Verification items for the finished model (mm, model axes). Give positions to 0.01 mm unless a question says otherwise; leave off trailing zeros. Loops run counter-clockwise (first coordinate to the right, second up) from the corner with the lowest first, then second, coordinate; pieces in that order, holes last. Notation, with made-up numbers: (51, -1) - (102, -1) arc R29 ccw to (102, 29) - close; hole circle Ø3 at (44.25, 49.25). An arc over 180 degrees is marked (long way). One line per question, with ' | ' between items. Start each with the question number.
1. Section check B-B, the plane y = 119.25. Enter the section's corners in (x, z) (3 decimals), then the cut area to 3 significant figures.
2. Thickness scan on line 1 along X through (y, z) = (122.25, 275) (3 decimals); line 2 along Z through (x, y) = (2300, 122) (3 decimals); line 3 along X through (y, z) = (123.5, 283). Record the ranges inside material, lowest first. Write a range as from..to.
3. Section check A-A, the plane z = 275. Enter the section's corners in (x, y) (3 decimals).
4. Section check C-C, the plane x = 2600. Enter the section's corners in (y, z) (3 decimals), then the cut area to 3 significant figures.
from build123d import *

# Parameters (mm, degrees)
BOSS_EXTRUDE1_DEPTH      = 50.8
BOSS_EXTRUDE1_DEPTH_BACK = 38.1
SKETCH2_W                = 381
SKETCH2_H                = 12.7
SKETCH3_W                = 12.7
SKETCH3_H                = 44.45
CUT_EXTRUDE1_DEPTH       = 2664.230012597
CAVITY1_START            = 115.8
CAVITY1_OUTLINE_R        = 12.7
CAVITY1_DEPTH            = 12.7
MOVE_FACE_HOLES_BY       = 0.635
MOVE_FACE_HOLES_2_BY     = 0.635
MOVE_FACE2_BY            = 0.762
MOVE_FACE2_2_BY          = 0.762
MOVE_FACE2_3_BY          = 0.762
SLOT_FILLET_R            = 3.175


# Read off the part's stored shape, not the designer's step: Cavity1
with BuildPart() as part:
    # Sketch2 → Boss-Extrude1 (new, two sides: drawn at the far end of the back side and taken through both)
    with BuildSketch(Plane.XY.offset(287.7).offset(-BOSS_EXTRUDE1_DEPTH_BACK)):
        with Locations((2451.1, 122.15)):
            Rectangle(SKETCH2_W, SKETCH2_H)
    extrude(amount=BOSS_EXTRUDE1_DEPTH + BOSS_EXTRUDE1_DEPTH_BACK)

    # Sketch3 → Cut-Extrude1 (cut, through all)
    with BuildSketch(Plane(origin=(0, 128.5, 0), x_dir=(1, 0, 0), z_dir=(0, 1, 0))):
        with Locations((2470.15, -271.825)):
            Rectangle(SKETCH3_W, SKETCH3_H)
    extrude(amount=-CUT_EXTRUDE1_DEPTH, mode=Mode.SUBTRACT)

    # Cavity1 outline → Cavity1 (cut)
    with BuildSketch(Plane(origin=(0, 0, 0), x_dir=(1, 0, 0), z_dir=(0, 1, 0)).offset(CAVITY1_START)):
        with Locations((2300, -275)):
            Circle(CAVITY1_OUTLINE_R)
        with Locations((2600, -275)):
            Circle(CAVITY1_OUTLINE_R)
    extrude(amount=CAVITY1_DEPTH, mode=Mode.SUBTRACT)

    # Move Face Holes: a curved face moved outward by 0.635
    add(Solid.thicken(part.faces().sort_by_distance((2587.3, 122.15, 275))[0], MOVE_FACE_HOLES_BY))

    # Move Face Holes 2: a curved face moved outward by 0.635
    add(Solid.thicken(part.faces().sort_by_distance((2287.3, 122.15, 275))[0], MOVE_FACE_HOLES_2_BY))

    # Move Face2: a face moved inward by 0.762
    extrude(part.faces().sort_by_distance((2470.15, 122.15, 294.05))[0], amount=MOVE_FACE2_BY, dir=(0, 0, 1), mode=Mode.SUBTRACT)

    # Move Face2 2: a face moved inward by 0.762
    extrude(part.faces().sort_by_distance((2476.5, 122.15, 271.825))[0], amount=MOVE_FACE2_2_BY, dir=(1, 0, 0), mode=Mode.SUBTRACT)

    # Move Face2 3: a face moved inward by 0.762
    extrude(part.faces().sort_by_distance((2463.8, 122.15, 271.825))[0], amount=MOVE_FACE2_3_BY, dir=(-1, 0, 0), mode=Mode.SUBTRACT)

    # Slot Fillet
    slot_fillet_edges = [part.edges().sort_by_distance(p)[0] for p in [
        (2477.262, 122.15, 294.812),
        (2463.038, 122.15, 294.812),
    ]]
    fillet(slot_fillet_edges, radius=SLOT_FILLET_R)


solid = part.part
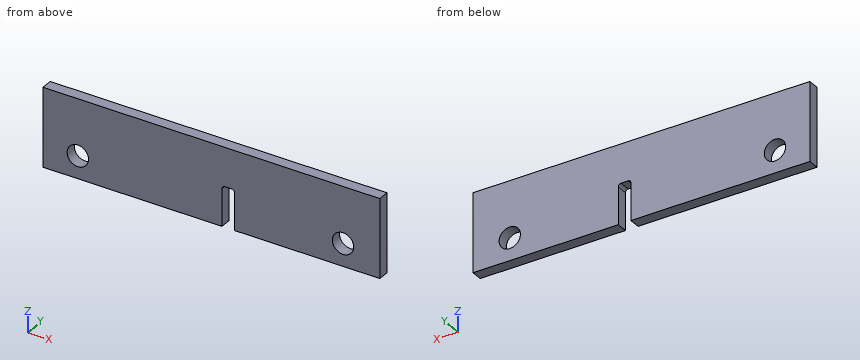
Results list:
1) outline: (2260.6, 249.6) - (2463.038, 249.6) - (2463.038, 291.637) arc R3.175 cw to (2466.213, 294.812) - (2474.087, 294.812) arc R3.175 cw to (2477.262, 291.637) - (2477.262, 249.6) - (2641.6, 249.6) - (2641.6, 338.5) - (2260.6, 338.5) - close; hole circle Ø24.13 at (2300, 275); hole circle Ø24.13 at (2600, 275) | area: 32,300 mm²
2) line 1: 2260.6..2287.935, 2312.065..2463.038, 2477.262..2587.935, 2612.065..2641.6 | line 2: 249.6..262.935, 287.065..338.5 | line 3: 2260.6..2290.97, 2309.03..2463.04, 2477.26..2590.97, 2609.03..2641.6
3) outline: (2260.6, 115.8) - (2287.935, 115.8) - (2287.935, 128.5) - (2260.6, 128.5) - close; (2312.065, 115.8) - (2463.038, 115.8) - (2463.038, 128.5) - (2312.065, 128.5) - close; (2477.262, 115.8) - (2587.935, 115.8) - (2587.935, 128.5) - (2477.262, 128.5) - close; (2612.065, 115.8) - (2641.6, 115.8) - (2641.6, 128.5) - (2612.065, 128.5) - close
4) outline: (115.8, 249.6) - (128.5, 249.6) - (128.5, 262.935) - (115.8, 262.935) - close; (115.8, 287.065) - (128.5, 287.065) - (128.5, 338.5) - (115.8, 338.5) - close | area: 823 mm²
